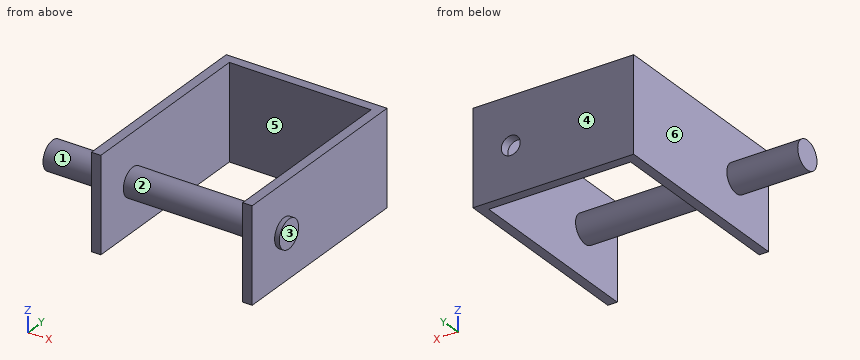
from build123d import *

# Parameters (mm, degrees)
EXTRUDE_1_DEPTH      = 20
SKETCH_3_R           = 3
EXTRUDE_2_DEPTH      = 15
EXTRUDE_2_DEPTH_BACK = 35
SKETCH_4_R           = 2
CUT_EXTRUDE_1_DEPTH  = 2


with BuildPart() as part:
    # 草图1 → 凸台-拉伸1 (new body)
    with BuildSketch(Plane.XY):
        Polygon((-38.9636651, 28.845358616), (-38.9636651, -11.154641384), (-36.9636651, -11.154641384), (-36.9636651, 28.845358616), (-6.9636651, 28.845358616), (-6.9636651, -11.154641384), (-4.9636651, -11.154641384), (-4.9636651, 30.845358616), (-38.9636651, 30.845358616), align=None)
    extrude(amount=EXTRUDE_1_DEPTH)

    # 草图3 → 凸台-拉伸2 (add, two sides)
    with BuildSketch(Plane.ZY.offset(38.9636651)) as extrude_2_sk:
        with Locations((10, -1.154641384)):
            Circle(SKETCH_3_R)
    extrude(amount=EXTRUDE_2_DEPTH)
    extrude(extrude_2_sk.sketch, amount=-EXTRUDE_2_DEPTH_BACK)

    # 草图4 → 切除-拉伸1 (cut)
    with BuildSketch(Plane(origin=(0, 30.845358616, 0), x_dir=(1, 0, 0), z_dir=(0, 1, 0))):
        with Locations((-12.9636651, -10)):
            Circle(SKETCH_4_R)
    extrude(amount=-CUT_EXTRUDE_1_DEPTH, mode=Mode.SUBTRACT)


solid = part.part
Check sheet for the modelled part. Datum: model origin and axes. Units: mm. Face numbers are marked on the shaded views. A direction names the side the tool comes from. Round coordinates to 2 decimals unless told otherwise and drop trailing zeros. Write each loop counter-clockwise with the first axis right and the second up, starting at its lowest first coordinate (ties: lowest second). Pieces come first, ordered by that corner, then holes. Notation, with made-up numbers: (64, 75.25) - (93, 75.25) arc R23 ccw to (93, 96.25) - close; hole circle Ø6 at (-6.5, 70.25). An arc over 180 degrees is marked (long way). Return JSON: item names as keys, results as strings.
Q1. Cross-section at B-B (z = 10). Record the boundary of the cut face in (x, y), then the cut area to 3 significant figures.
Returned:
{"outline": "(-53.96, -4.15) - (-38.96, -4.15) - (-38.96, -11.15) - (-36.96, -11.15) - (-36.96, -4.15) - (-6.96, -4.15) - (-6.96, -11.15) - (-4.96, -11.15) - (-4.96, -4.15) - (-3.96, -4.15) - (-3.96, 1.85) - (-4.96, 1.85) - (-4.96, 30.85) - (-10.96, 30.85) - (-10.96, 28.85) - (-6.96, 28.85) - (-6.96, 1.85) - (-36.96, 1.85) - (-36.96, 28.85) - (-14.96, 28.85) - (-14.96, 30.85) - (-38.96, 30.85) - (-38.96, 1.85) - (-53.96, 1.85) - close", "area": "496 mm²"}
Q2. Cross-section at C-C (x = -12). Record the boundary of the cut face in (y, z).
Returned:
{"outline": "circle Ø6 at (-1.15, 10); (28.85, 0) - (30.85, 0) - (30.85, 8.25) - (28.85, 8.25) - close; (28.85, 11.75) - (30.85, 11.75) - (30.85, 20) - (28.85, 20) - close"}
Q3. Cross-section at D-D (x = -28). Record the boundary of the cut face in (y, z).
Returned:
{"outline": "circle Ø6 at (-1.15, 10); (28.85, 0) - (30.85, 0) - (30.85, 20) - (28.85, 20) - close"}
Q4. Depth check by flat-ended pin: P1, Ø3, axis at x = -24.5, y = 1, coming from the +Z side; P2, Ø1.5, axis at x = -46, y = -4, coming from the -Z side; P3, Ø5, axis at x = -19.5, z = 6.5, coming from the -Y side. Enter the tip coordinate at first touch or a pass-through.
Returned:
{"P1": "stops at z = 12.93", "P2": "stops at z = 7.85", "P3": "stops at y = -3.98"}
Q5. Access from +Z, -Z, +X, -X, +Y, -Y to the whole of each face (thin tool, end or side, straight path). Record for the marked faces 1, 2 and 3.
Returned:
{"face 1": "-X", "face 2": "none", "face 3": "+Z, -Z, +X, +Y, -Y"}
Q6. Draft check along X on the marked faces 4, 5 and 6. Enter one of: released by +X, released by -X, zero draft, split by the parting line, or undercut.
Returned:
{"face 4": "zero draft", "face 5": "undercut", "face 6": "released by -X"}
Q7. Scan lines: L1, parallel to X at y = 29.6, z = 10; L2, parallel to X at y = 9, z = 16.5; L3, parallel to Y at x = -17, z = 1. Record each from-to range of solid material in increasing order. Write a range as from..to.
Returned:
{"L1": "x = -38.96..-14.96, -10.96..-4.96", "L2": "x = -38.96..-36.96, -6.96..-4.96", "L3": "y = 28.85..30.85"}
Q8. Cross-section at A-A (y = 18). Record the boundary of the cut face in (x, z).
Returned:
{"outline": "(-38.96, 0) - (-36.96, 0) - (-36.96, 20) - (-38.96, 20) - close; (-6.96, 0) - (-4.96, 0) - (-4.96, 20) - (-6.96, 20) - close"}
